```python
from build123d import *

# Parameters (mm, degrees)
F0_W      = 342.9
F0_H      = 177.8
F0_W_2    = 228.6
F0_H_2    = 215.9
F1_DEPTH  = 25.4
F2_W      = 304.8
F2_H      = 12.7
F3_DEPTH  = 12.7
F4_W      = 304.8
F4_H      = 12.7
F5_DEPTH  = 12.7
F6_R      = 12.7
F7_DEPTH  = 25.4
F9_DEPTH  = 12.7
F11_DEPTH = 12.7
F12_W     = 317.5
F12_H     = 12.7
F13_DEPTH = 12.7


with BuildPart() as f1:
    # F0 (on Front) → F1 (new body)
    with BuildSketch(Plane.XZ):
        with Locations((171.45, 88.9)):
            Rectangle(F0_W, F0_H)
        Polygon((0, 241.3), (0, 177.8), (342.9, 177.8), (342.9, 241.3), (285.75, 241.3), (57.15, 241.3), align=None)
        with Locations((171.45, 349.25)):
            Rectangle(F0_W_2, F0_H_2)
    extrude(amount=F1_DEPTH)

    # F2 (on face) → F3 (cut)
    with BuildSketch(Plane.XZ.offset(25.4)):
        with Locations((177.8, 12.7)):
            Rectangle(F2_W, F2_H)
    extrude(amount=-F3_DEPTH, mode=Mode.SUBTRACT)

    # F4 (on face) → F5 (cut)
    with BuildSketch(Plane.XZ.offset(25.4)):
        with Locations((177.8, -12.7)):
            Rectangle(F4_W, F4_H)
    extrude(amount=-F5_DEPTH, mode=Mode.SUBTRACT)

    # F6 (on face) → F7 (cut)
    with BuildSketch(Plane(origin=(0, 0, 0), x_dir=(-1, 0, 0), z_dir=(0, 1, 0))):
        with Locations((-63.5, 38.1)):
            Circle(F6_R)
    extrude(amount=-F7_DEPTH, mode=Mode.SUBTRACT)

    # F8 (on face) → F9 (cut)
    with BuildSketch(Plane.XZ.offset(25.4)):
        Polygon((323.85, 44.45), (330.2, 44.45), (336.55, 44.45), (336.55, 133.35), (323.85, 133.35), align=None)
    extrude(amount=-F9_DEPTH, mode=Mode.SUBTRACT)

    # F10 (on face) → F11 (cut)
    with BuildSketch(Plane.XZ.offset(25.4)):
        Polygon((76.2, 438.15), (76.2, 457.2), (57.15, 457.2), (57.15, 241.3), (76.2, 241.3), align=None)
        Polygon((285.75, 241.3), (285.75, 457.2), (266.7, 457.2), (266.7, 438.15), (266.7, 241.3), align=None)
    extrude(amount=-F11_DEPTH, mode=Mode.SUBTRACT)

    # F12 (on face) → F13 (cut)
    with BuildSketch(Plane.XZ.offset(25.4)):
        with Locations((171.45, 209.55)):
            Rectangle(F12_W, F12_H)
        with Locations((171.45, 184.15)):
            Rectangle(F12_W, F12_H)
    extrude(amount=-F13_DEPTH, mode=Mode.SUBTRACT)


solid = f1.part
```
Geometry check sheet. Reference: the model listing, model coordinates, mm. A direction names the side the tool comes from. Give positions to 0.01 mm unless a question says otherwise; leave off trailing zeros. Loops run counter-clockwise (first coordinate to the right, second up) from the corner with the lowest first, then second, coordinate; pieces in that order, holes last. Notation, with made-up numbers: (43.25, 63.25) - (92.25, 63.25) arc R24 ccw to (92.25, 90.25) - close; hole circle Ø1 at (15, -19.75). An arc over 180 degrees is marked (long way). Use CSV: the item, a comma, the result in double quotes. Start each with the question number.
Q1. Go/stop test with flat-tipped pins: pin 1 Ø6.5 at (y, z) = (-9.5, 397) entering from +X; pin 2 Ø1 at (y, z) = (-19.5, 307) entering from -X; pin 3 Ø4 at (x, y) = (328.5, -16) entering from +Z. Record where each tip stops, or that it passes through.
Q2. Section check A-A, the plane z = 38.1. Record the cut outline in (x, y), and give its area (3 significant figures).
Q3. Section check D-D, the plane x = 63.5. Record the cut outline in (y, z).
Q4. Section check B-B, the plane y = -19.75. Record the cut outline in (x, z).
Q5. Section check C-C, the plane x = 186. Record the cut outline in (y, z), and give its area (3 significant figures).
Q6. Scan lines: probe 1 along Z at (x, y) = (97.5, -21); probe 2 along Z at (x, y) = (63.5, -20); probe 3 along Z at (x, y) = (63.5, -7). Record each from-to range of solid material in increasing order. Write a range as from..to.
Q7. Release check for a two-part mould opening along Z. For faces 1 (the face through (176, -12.7, 13)), 2 (the face through (169, -13, 0)), 3 (the face through (336.55, -19, 88)), 4 (the face through (57.15, -6, 348)) record: +Z half, -Z half, draft (parallel to the pull), parting line (faces both ways), or undercut.
Q8. Access from +Z, -Z, +X, -X, +Y, -Y to the whole of each face (thin tool, end or side, straight path). Record for faces 5 (the face through (176, -19, 19.05)), 6 (the face through (276, -12.7, 351)), 7 (the face through (56.673, -12.522, 48.809)).
Findings below:
1,pin 1,"stops at x = 285.75"
1,pin 2,"stops at x = 76.2"
1,pin 3,"stops at z = 241.3"
2,outline,"(0, -25.4) - (50.8, -25.4) - (50.8, 0) - (0, 0) - close; (76.2, -25.4) - (342.9, -25.4) - (342.9, 0) - (76.2, 0) - close"
2,area,"8,060 mm^2"
3,outline,"(-25.4, 0) - (0, 0) - (0, 25.4) - (-25.4, 25.4) - (-25.4, 19.05) - (-12.7, 19.05) - (-12.7, 6.35) - (-25.4, 6.35) - close; (-25.4, 50.8) - (0, 50.8) - (0, 457.2) - (-12.7, 457.2) - (-12.7, 241.3) - (-25.4, 241.3) - (-25.4, 215.9) - (-12.7, 215.9) - (-12.7, 203.2) - (-25.4, 203.2) - (-25.4, 190.5) - (-12.7, 190.5) - (-12.7, 177.8) - (-25.4, 177.8) - close"
4,outline,"(0, 0) - (342.9, 0) - (342.9, 241.3) - (266.7, 241.3) - (266.7, 457.2) - (76.2, 457.2) - (76.2, 241.3) - (0, 241.3) - close; hole (12.7, 177.8) - (330.2, 177.8) - (330.2, 190.5) - (12.7, 190.5) - close; hole (12.7, 203.2) - (330.2, 203.2) - (330.2, 215.9) - (12.7, 215.9) - close; hole (25.4, 6.35) - (330.2, 6.35) - (330.2, 19.05) - (25.4, 19.05) - close; hole circle Ø25.4 at (63.5, 38.1); hole (323.85, 44.45) - (336.55, 44.45) - (336.55, 133.35) - (323.85, 133.35) - close"
5,outline,"(-25.4, 0) - (0, 0) - (0, 457.2) - (-25.4, 457.2) - (-25.4, 215.9) - (-12.7, 215.9) - (-12.7, 203.2) - (-25.4, 203.2) - (-25.4, 190.5) - (-12.7, 190.5) - (-12.7, 177.8) - (-25.4, 177.8) - (-25.4, 19.05) - (-12.7, 19.05) - (-12.7, 6.35) - (-25.4, 6.35) - close"
5,area,"11,100 mm^2"
6,probe 1,"z = 0..6.35, 19.05..177.8, 190.5..203.2, 215.9..457.2"
6,probe 2,"z = 0..6.35, 19.05..25.4, 50.8..177.8, 190.5..203.2, 215.9..241.3"
6,probe 3,"z = 0..25.4, 50.8..457.2"
7,face 1,"undercut"
7,face 2,"-Z half"
7,face 3,"undercut"
7,face 4,"draft"
8,face 5,"-Y"
8,face 6,"+Z, +X, -Y"
8,face 7,"+Y, -Y"
